Part print with two shaded views. Sizes in mm from the minimum x, y, z corner. A direction names the side the tool comes from. Round coordinates to 2 decimals unless told otherwise and drop trailing zeros. Write each loop counter-clockwise with the first axis right and the second up, starting at its lowest first coordinate (ties: lowest second). Pieces come first, ordered by that corner, then holes. Notation, with made-up numbers: (-12.5, -37.75) -> (1.5, -37.75) arc R6 ccw to (1.5, -33.75) -> close; hole circle Ø9 at (3.25, 26.25). An arc over 180 degrees is marked (long way). Put each result on its own line as item: value. Start each with the question number.
1. Drill centre lines: line 1 (Y direction, x = 53, z = 28.5); line 2 (Z direction, x = 55, y = 38); line 3 (X direction, y = 91, z = 16.5). Where is each one in solid material? Low to high. Write a range as from..to.
2. 3-axis set-ups, long thin cutter, end or side, ignore diameter. For the marked faces 4 and 5: which of +Z, -Z, +X, -X, +Y, -Y reach the whole face in a straight line?
3. Saw through at A-A on z = 21. List the corners of the cut face in (x, y).
4. Flat gauge pin, fed straight in: P1, Ø6, axis at y = 51, z = 22, coming from the -X side. Where does the tip first touch, or does it go through?
5. Saw through at C-C on y = 64.5. List the corners of the cut face in (x, z).
6. Saw through at B-B on x = 60. List the corners of the cut face in (y, z).
7. Pull direction Y, two halves, no side cores. Call the marked faces 1, 2 and 3: pulls with the +Y half, pulls with the -Y half, needs draft (parallel to the pull), parting line crosses it, or undercut.
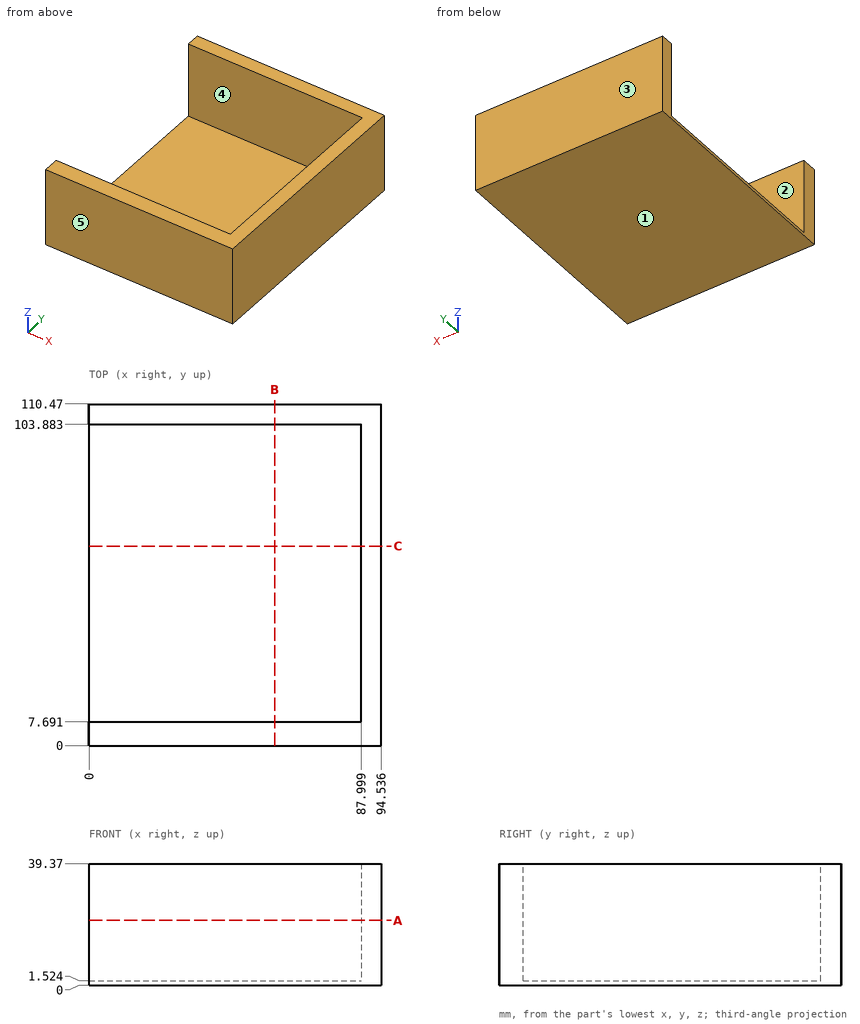
Return value:
1. line 1: y = 0..7.69, 103.88..110.47
1. line 2: z = 0..1.52
1. line 3: x = 88..94.54
2. face 4: +Z, -X
2. face 5: +Z, -Z, +X, -X, -Y
3. outline: (0, 0) -> (94.54, 0) -> (94.54, 110.47) -> (0, 110.47) -> (0, 103.88) -> (88, 103.88) -> (88, 7.69) -> (0, 7.69) -> close
4. P1: stops at x = 88
5. outline: (0, 0) -> (94.54, 0) -> (94.54, 39.37) -> (88, 39.37) -> (88, 1.52) -> (0, 1.52) -> close
6. outline: (0, 0) -> (110.47, 0) -> (110.47, 39.37) -> (103.88, 39.37) -> (103.88, 1.52) -> (7.69, 1.52) -> (7.69, 39.37) -> (0, 39.37) -> close
7. face 1: needs draft
7. face 2: undercut
7. face 3: pulls with the +Y half
